Verification items for this drawing (mm, ordinates from the low corner). Round coordinates to 2 decimals unless told otherwise and drop trailing zeros. Order: outer loops, then holes, each group sorted by start corner. A loop starts at its lowest first (then second) coordinate and runs counter-clockwise, first axis right, second up.
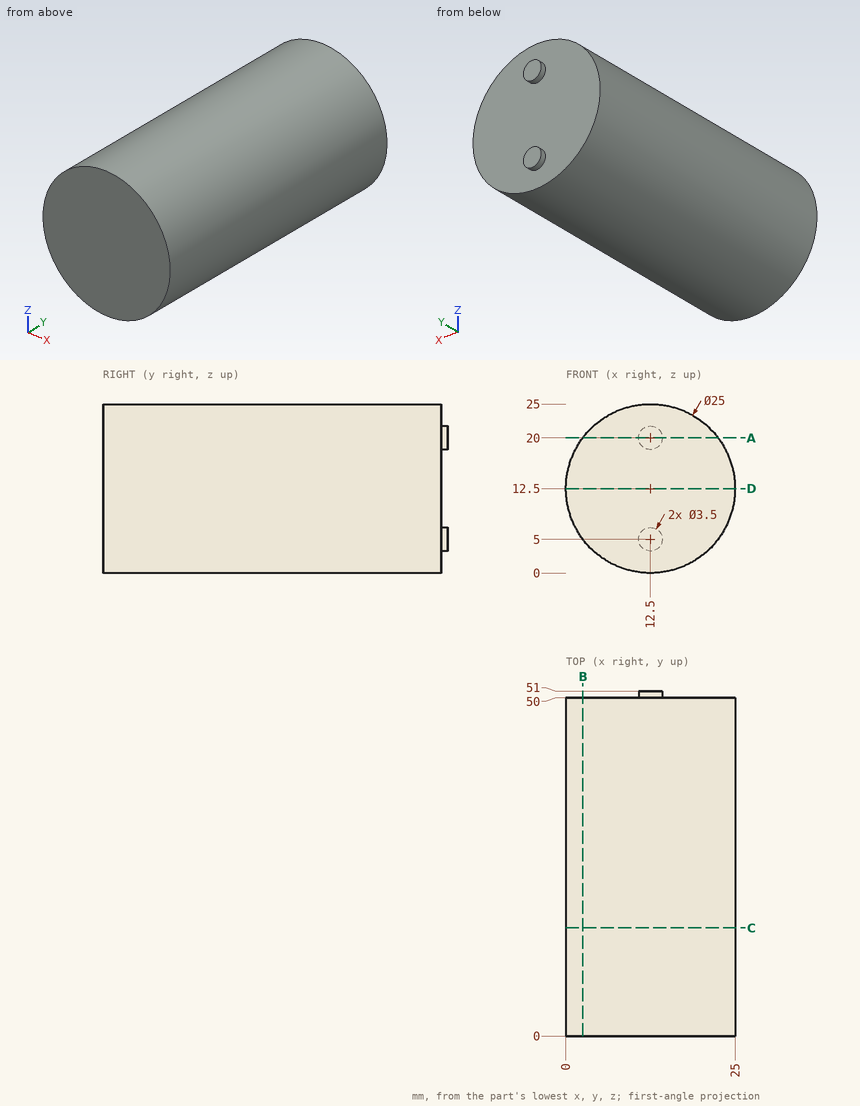
Item 1: Sectioned sample at A-A (z = 20). Record the cut outline in (x, y), and give its area (3 significant figures).
Answer:
outline: (2.5, 0) - (22.5, 0) - (22.5, 50) - (14.25, 50) - (14.25, 51) - (10.75, 51) - (10.75, 50) - (2.5, 50) - close
area: 1,000 mm2
Item 2: Sectioned sample at D-D (z = 12.5). Record the cut outline in (x, y), and give its area (3 significant figures).
Answer:
outline: (0, 0) - (25, 0) - (25, 50) - (0, 50) - close
area: 1,250 mm2
Item 3: Go/stop test with flat-tipped pins: P1, Ø5, axis at x = 6, y = 10, coming from the +Z side; P2, Ø8, axis at x = 19, y = 35.5, coming from the +Z side; P3, Ø6, axis at x = 22.5, z = 9, coming from the +Y side. Record where each tip stops, or that it passes through.
Answer:
P1: stops at z = 24.34
P2: stops at z = 24.75
P3: stops at y = 50
Item 4: Sectioned sample at C-C (y = 16). Record the cut outline in (x, z), and give its area (3 significant figures).
Answer:
outline: circle Ø25 at (12.5, 12.5)
area: 491 mm2
Item 5: Sectioned sample at B-B (x = 2.5). Record the cut outline in (y, z).
Answer:
outline: (0, 5) - (50, 5) - (50, 20) - (0, 20) - close
Item 6: Scan lines: line 1 along X through (y, z) = (31, 12); line 2 along Y through (x, z) = (12.5, 17.75); line 3 along Z through (x, y) = (16.5, 4). Record each from-to range of solid material in increasing order.
Answer:
line 1: x = 0.01 to 24.99
line 2: y = 0 to 50
line 3: z = 0.66 to 24.34
